```python
from build123d import *

# Parameters (mm, degrees)
SKETCH_1_R      = 25
EXTRUDE_1_DEPTH = 80
SKETCH_2_W      = 30
SKETCH_2_H      = 30
EXTRUDE_2_DEPTH = 230


with BuildPart() as part:
    # 草图1 → 凸台-拉伸1 (new body)
    with BuildSketch(Plane(origin=(0, 0, 0), x_dir=(1, 0, 0), z_dir=(0, 1, 0))):
        Circle(SKETCH_1_R)
    extrude(amount=EXTRUDE_1_DEPTH)

    # 草图2 → 凸台-拉伸2 (add)
    with BuildSketch(Plane(origin=(0, 80, 0), x_dir=(1, 0, 0), z_dir=(0, 1, 0))):
        Rectangle(SKETCH_2_W, SKETCH_2_H)
    extrude(amount=EXTRUDE_2_DEPTH)


solid = part.part
```
Read the model definition and answer for the solid it produces. Units are mm, in the model's axes. A direction names the side the tool comes from. Round coordinates to 2 decimals unless told otherwise and drop trailing zeros. Write each loop counter-clockwise with the first axis right and the second up, starting at its lowest first coordinate (ties: lowest second). Pieces come first, ordered by that corner, then holes. Notation, with made-up numbers: (45.5, 67) - (63.5, 67) arc R17 ccw to (63.5, 80) - close; hole circle Ø1 at (-7.5, -30). An arc over 180 degrees is marked (long way). One line per item, written item: value.
Q1. Find section D-D (x = 19). Determine the outline of the cut face in (y, z), and give its area (3 significant figures).
The answers:
outline: (0, -16.25) - (80, -16.25) - (80, 16.25) - (0, 16.25) - close
area: 2,600 mm2
Q2. Find section C-C (y = 30). Determine the outline of the cut face in (x, z).
The answers:
outline: circle Ø50 at (0, 0)
Q3. Which of the six approach directions +Z, -Z, +X, -X, +Y, -Y give full straight-line access (tool end or side, diameter ignored) to faces 1 (the flat face through (0, 0, 0)), 2 (the flat face through (15, 193, 0)), 3 (the flat face through (-15, 193, 0)), 4 (the flat face through (0, 193, 15)), 5 (the flat face through (0, 193, -15))?
The answers:
face 1: +Z, -Z, +X, -X, -Y
face 2: +Z, -Z, +X, +Y
face 3: +Z, -Z, -X, +Y
face 4: +Z, +X, -X, +Y
face 5: -Z, +X, -X, +Y
Q4. Straight lines are drawn through the part: line 1 (Z direction, x = 11.5, y = 270.5); line 2 (Y direction, x = -0.5, z = 22). For each, find the intervals that lie inside material, in ascending order. Write a range as from..to.
The answers:
line 1: z = -15..15
line 2: y = 0..80
Q5. Find section B-B (x = 0). Determine the outline of the cut face in (y, z), and give its area (3 significant figures).
The answers:
outline: (0, -25) - (80, -25) - (80, -15) - (310, -15) - (310, 15) - (80, 15) - (80, 25) - (0, 25) - close
area: 10,900 mm2
Q6. Find section A-A (z = 0). Determine the outline of the cut face in (x, y), and give its area (3 significant figures).
The answers:
outline: (-25, 0) - (25, 0) - (25, 80) - (15, 80) - (15, 310) - (-15, 310) - (-15, 80) - (-25, 80) - close
area: 10,900 mm2
Q7. Each of these flat-tipped pins is pushed along its axis until it touches: P1, Ø24, axis at y = 138.5, z = -7.5, coming from the +X side; P2, Ø9, axis at x = -0.5, y = 196, coming from the +Z side; P3, Ø15, axis at y = 161, z = -2, coming from the -X side. Where does it stop, or does it pass through?
The answers:
P1: stops at x = 15
P2: stops at z = 15
P3: stops at x = -15
